from build123d import *

# Parameters (mm, degrees)
SKETCH_1_W      = 200
SKETCH_1_H      = 150
SKETCH_1_R      = 2.5
EXTRUDE_1_DEPTH = 1.5


with BuildPart() as part:
    # 草图1 → 凸台-拉伸1 (new body)
    with BuildSketch(Plane.XY):
        Rectangle(SKETCH_1_W, SKETCH_1_H)
        with Locations((-82, 0)):
            Circle(SKETCH_1_R, mode=Mode.SUBTRACT)
        with Locations((-59, 0)):
            Circle(SKETCH_1_R, mode=Mode.SUBTRACT)
        with Locations(Location((59, 0, 0), (0, 0, 180))):
            Circle(SKETCH_1_R, mode=Mode.SUBTRACT)
        with Locations(Location((82, 0, 0), (0, 0, 180))):
            Circle(SKETCH_1_R, mode=Mode.SUBTRACT)
        with Locations((-35, -34)):
            Circle(SKETCH_1_R, mode=Mode.SUBTRACT)
        with Locations((-35, -57)):
            Circle(SKETCH_1_R, mode=Mode.SUBTRACT)
        with Locations(Location((35, -57, 0), (0, 0, 180))):
            Circle(SKETCH_1_R, mode=Mode.SUBTRACT)
        with Locations(Location((35, -34, 0), (0, 0, 180))):
            Circle(SKETCH_1_R, mode=Mode.SUBTRACT)
        with Locations((35, 57)):
            Circle(SKETCH_1_R, mode=Mode.SUBTRACT)
        with Locations((35, 34)):
            Circle(SKETCH_1_R, mode=Mode.SUBTRACT)
        with Locations(Location((-35, 57, 0), (0, 0, 180))):
            Circle(SKETCH_1_R, mode=Mode.SUBTRACT)
        with Locations(Location((-35, 34, 0), (0, 0, 180))):
            Circle(SKETCH_1_R, mode=Mode.SUBTRACT)
    extrude(amount=EXTRUDE_1_DEPTH)


solid = part.part
The listing builds one solid part. Answer for the finished solid, in the listing's coordinates (mm). Round coordinates to 2 decimals unless told otherwise and drop trailing zeros. Write each loop counter-clockwise with the first axis right and the second up, starting at its lowest first coordinate (ties: lowest second). Pieces come first, ordered by that corner, then holes. Notation, with made-up numbers: (73.25, 7) - (117.25, 7) arc R27 cw to (117.25, 25) - close; hole circle Ø3 at (-3, 62.25). An arc over 180 degrees is marked (long way). Use a Markdown table: item, result. Add a question column.
1. The part is cut by section A-A (y = 0). Write down the section's boundary in (x, z).
2. For a pull along X with two mould halves and no side action, classify faces 1 (the face through (-1, 1, 0)), 2 (the face through (-56.69, -0.96, 0.74)) as +X half, -X half, draft (parallel to the pull), parting line (faces both ways), or undercut.
3. Consider line 1 (Y direction, x = -35, z = 0.75); line 2 (Y direction, x = 59, z = 0.55); line 3 (X direction, y = -55, z = 0.3). Determine where each line is inside the solid, lowest interval first.
4. The part is cut by section C-C (y = 57). Write down the section's boundary in (x, z), and give its area (3 significant figures).
5. The part is cut by section B-B (x = 82). Write down the section's boundary in (y, z).
6. The part is cut by section D-D (x = -35). Write down the section's boundary in (y, z), and give its area (3 significant figures).
Reported:
| question | item | result |
|---|---|---|
| 1 | outline | (-100, 0) - (-84.5, 0) - (-84.5, 1.5) - (-100, 1.5) - close; (-79.5, 0) - (-61.5, 0) - (-61.5, 1.5) - (-79.5, 1.5) - close; (-56.5, 0) - (56.5, 0) - (56.5, 1.5) - (-56.5, 1.5) - close; (61.5, 0) - (79.5, 0) - (79.5, 1.5) - (61.5, 1.5) - close; (84.5, 0) - (100, 0) - (100, 1.5) - (84.5, 1.5) - close |
| 2 | face 1 | draft |
| 2 | face 2 | undercut |
| 3 | line 1 | -75 to -59.5, -54.5 to -36.5, -31.5 to 31.5, 36.5 to 54.5, 59.5 to 75 |
| 3 | line 2 | -75 to -2.5, 2.5 to 75 |
| 3 | line 3 | -100 to -36.5, -33.5 to 33.5, 36.5 to 100 |
| 4 | outline | (-100, 0) - (-37.5, 0) - (-37.5, 1.5) - (-100, 1.5) - close; (-32.5, 0) - (32.5, 0) - (32.5, 1.5) - (-32.5, 1.5) - close; (37.5, 0) - (100, 0) - (100, 1.5) - (37.5, 1.5) - close |
| 4 | area | 285 mm^2 |
| 5 | outline | (-75, 0) - (-2.5, 0) - (-2.5, 1.5) - (-75, 1.5) - close; (2.5, 0) - (75, 0) - (75, 1.5) - (2.5, 1.5) - close |
| 6 | outline | (-75, 0) - (-59.5, 0) - (-59.5, 1.5) - (-75, 1.5) - close; (-54.5, 0) - (-36.5, 0) - (-36.5, 1.5) - (-54.5, 1.5) - close; (-31.5, 0) - (31.5, 0) - (31.5, 1.5) - (-31.5, 1.5) - close; (36.5, 0) - (54.5, 0) - (54.5, 1.5) - (36.5, 1.5) - close; (59.5, 0) - (75, 0) - (75, 1.5) - (59.5, 1.5) - close |
| 6 | area | 195 mm^2 |
